```python
from build123d import *

# Parameters (mm, degrees)
IZIM1_R                     = 17.5
IZIM1_R_2                   = 17
Y_KSEKLIK_EKSTR_ZYON1_DEPTH = 9
KAL_NLA_T_R1_OUTLINE_R      = 17
KAL_NLA_T_R1_DEPTH          = 2
IZIM2_R                     = 2.9
KES_EKSTR_ZYON1_DEPTH       = 9
KES_EKSTR_ZYON5_DEPTH       = 43.349734356
DAIRESEL_KAPLAMA1_COUNT     = 2
DAIRESEL_KAPLAMA1_ANGLE     = 90
IZIM4_R                     = 5.5
Y_KSEKLIK_EKSTR_ZYON2_DEPTH = 4.2
IZIM5_R                     = 2.5
Y_KSEKLIK_EKSTR_ZYON3_DEPTH = 11


# Read off the part's stored shape, not the designer's step: Kalınlaştır1
with BuildPart() as part:
    # Çizim1 → Yükseklik-Ekstrüzyon1 (new body)
    with BuildSketch(Plane(origin=(0, 0, 0), x_dir=(1, 0, 0), z_dir=(0, 1, 0))):
        with Locations(Location((0, 0, 0), (0, 0, 270))):
            Circle(IZIM1_R)
        with Locations(Location((0, 0, 0), (0, 0, 270))):
            Circle(IZIM1_R_2, mode=Mode.SUBTRACT)
    extrude(amount=Y_KSEKLIK_EKSTR_ZYON1_DEPTH)

    # Kalınlaştır1 outline → Kalınlaştır1 (add)
    with BuildSketch(Plane(origin=(0, 0, 0), x_dir=(1, 0, 0), z_dir=(0, 1, 0))):
        Circle(KAL_NLA_T_R1_OUTLINE_R)
    extrude(amount=KAL_NLA_T_R1_DEPTH)

    # Çizim2 → Kes-Ekstrüzyon1 (cut)
    with BuildSketch(Plane(origin=(0, 2, 0), x_dir=(1, 0, 0), z_dir=(0, 1, 0))):
        with Locations(Location((-9.5, 0, 0), (0, 0, 270))):
            Circle(IZIM2_R)
        with Locations(Location((0, 9.5, 0), (0, 0, 270))):
            Circle(IZIM2_R)
        with Locations(Location((9.5, 0, 0), (0, 0, 270))):
            Circle(IZIM2_R)
        with Locations(Location((0, -9.5, 0), (0, 0, 270))):
            Circle(IZIM2_R)
    extrude(amount=-KES_EKSTR_ZYON1_DEPTH, mode=Mode.SUBTRACT)

    # Çizim3 → Kes-Ekstrüzyon5 (cut, symmetric)
    with BuildSketch(Plane.ZY.offset(-20)):
        with BuildLine():
            Line((-5.5, 7), (5.5, 7))
            ThreePointArc((5.5, 7), (7, 5.5), (5.5, 4))
            Line((5.5, 4), (-5.5, 4))
            ThreePointArc((-5.5, 4), (-7, 5.5), (-5.5, 7))
        make_face()
    kes_ekstr_zyon5 = extrude(amount=KES_EKSTR_ZYON5_DEPTH, both=True, mode=Mode.SUBTRACT)

    # Dairesel Kaplama1: Kes-Ekstrüzyon5 ×2 about axis
    dairesel_kaplama1_axis = Axis((0, 2, 0), (0, 1, 0))
    for i in range(1, DAIRESEL_KAPLAMA1_COUNT):
        add(kes_ekstr_zyon5.rotate(dairesel_kaplama1_axis, i * DAIRESEL_KAPLAMA1_ANGLE / (DAIRESEL_KAPLAMA1_COUNT - 1)), mode=Mode.SUBTRACT)

    # Çizim4 → Yükseklik-Ekstrüzyon2 (add)
    with BuildSketch(Plane.XZ):
        with Locations(Location((0, 0, 0), (0, 0, 90))):
            Circle(IZIM4_R)
    extrude(amount=Y_KSEKLIK_EKSTR_ZYON2_DEPTH)

    # Çizim5 → Yükseklik-Ekstrüzyon3 (add)
    with BuildSketch(Plane.XZ.offset(4.2)):
        with Locations(Location((0, 0, 0), (0, 0, 270))):
            Circle(IZIM5_R)
    extrude(amount=Y_KSEKLIK_EKSTR_ZYON3_DEPTH)


solid = part.part
```
Build history of the part. All positions in model axes, mm. A direction names the side the tool comes from. Round coordinates to 2 decimals unless told otherwise and drop trailing zeros. Order: outer loops, then holes, each group sorted by start corner. A loop starts at its lowest first (then second) coordinate and runs counter-clockwise, first axis right, second up. Notation, with made-up numbers: (33.25, -8) -> (74.25, -8) arc R18 cw to (74.25, -4) -> close; hole circle Ø2 at (72.5, 81.5). An arc over 180 degrees is marked (long way). Answer in a Markdown table with one row per item.
1) Band-saw the part on B-B on y = 5.5. Give the cut face in (x, z).
Values:
| item | result |
|---|---|
| outline | (-16.04, -7) arc R17.5 ccw to (-7, -16.04) -> (-7, -15.49) arc R17 cw to (-15.49, -7) -> close; (-16.04, 7) -> (-15.49, 7) arc R17 cw to (-7, 15.49) -> (-7, 16.04) arc R17.5 ccw to start; (7, -16.04) arc R17.5 ccw to (16.04, -7) -> (15.49, -7) arc R17 cw to (7, -15.49) -> close; (7, 15.49) arc R17 cw to (15.49, 7) -> (16.04, 7) arc R17.5 ccw to (7, 16.04) -> close |
2) Mould opens along Y. For faces 6 (the cylindrical face through (0.1, 1, -12.4)), 7 (the flat face through (17, 9, -3)), 8 (the cylindrical face through (15.8, 5.5, 7)) say: released by +Y, released by -Y, zero draft, split by the parting line, or undercut.
Values:
| item | result |
|---|---|
| face 6 | zero draft |
| face 7 | released by +Y |
| face 8 | undercut |
3) Pin check, flat tips, straight feed: P1, Ø7.5, axis at x = 0, z = -9.5, coming from the +Y side; P2, Ø5, axis at x = 13.5, y = 5.5, coming from the +Z side; P3, Ø5, axis at x = 9.5, z = 0, coming from the -Y side; P4, Ø0.7, axis at x = 16.5, z = -1.5, coming from the -Y side. Stop position of each tip, or through.
Values:
| item | result |
|---|---|
| P1 | y = 2 |
| P2 | z = 13.61 |
| P3 | through |
| P4 | y = 0 |
4) Wall check: L1, parallel to X at y = 0.6, z = 0; L2, parallel to Y at x = 5.5, z = 15; L3, parallel to Z at x = 11.5, y = 4. Give the ranges that are in metal, low to high.
Values:
| item | result |
|---|---|
| L1 | -17.5 to -12.4, -6.6 to 6.6, 12.4 to 17.5 |
| L2 | 0 to 2 |
| L3 | -13.19 to -12.52, 12.52 to 13.19 |
5) Which spindle directions (+Z, -Z, +X, -X, +Y, -Y) get a long thin tool onto all of the face, cutting with end or side? Do faces 1 (the flat face through (0.1, 4, 17.3)), 2 (the cylindrical face through (-2.44, -9.62, 0.54)), 3 (the flat face through (17.3, 7, 0)), 4 (the cylindrical face through (7.735, 1.014, -2.301)), 5 (the cylindrical face through (-10.344, 5.451, -13.491)). Say none if no direction does.
Values:
| item | result |
|---|---|
| face 1 | +Z, -Z |
| face 2 | -Y |
| face 3 | +X, -X |
| face 4 | +Y, -Y |
| face 5 | +Y |
6) Band-saw the part on D-D on z = 10. Give the cut face in (x, y), and give its area (3 significant figures).
Values:
| item | result |
|---|---|
| outline | (-14.36, 0) -> (-2.86, 0) -> (-2.86, 2) -> (-13.75, 2) -> (-13.75, 9) -> (-14.36, 9) -> close; (2.86, 0) -> (14.36, 0) -> (14.36, 9) -> (13.75, 9) -> (13.75, 2) -> (2.86, 2) -> close |
| area | 54.6 mm2 |
7) Band-saw the part on C-C on x = -11. Give the cut face in (y, z), and give its area (3 significant figures).
Values:
| item | result |
|---|---|
| outline | (0, -13.61) -> (9, -13.61) -> (9, -12.96) -> (2, -12.96) -> (2, -2.48) -> (0, -2.48) -> close; (0, 2.48) -> (2, 2.48) -> (2, 12.96) -> (9, 12.96) -> (9, 13.61) -> (0, 13.61) -> close |
| area | 53.6 mm2 |
8) Band-saw the part on A-A on z = 0. Give the number of separate pieces and of enclosed holes in the cut face, and give its area (3 significant figures).
Values:
| item | result |
|---|---|
| separate pieces | 5 |
| enclosed holes | 0 |
| area | 152 mm2 |
